Study the drawing (mm; zero at the part's minimum x, y, z) and answer. Round coordinates to 2 decimals unless told otherwise and drop trailing zeros. Order: outer loops, then holes, each group sorted by start corner. A loop starts at its lowest first (then second) coordinate and runs counter-clockwise, first axis right, second up. Notation, with made-up numbers: (-38.5, -1) -> (-12.5, -1) arc R32 ccw to (-12.5, 36) -> close; hole circle Ø8 at (19.25, 7). An arc over 180 degrees is marked (long way). Use one line per item in the form item = value.
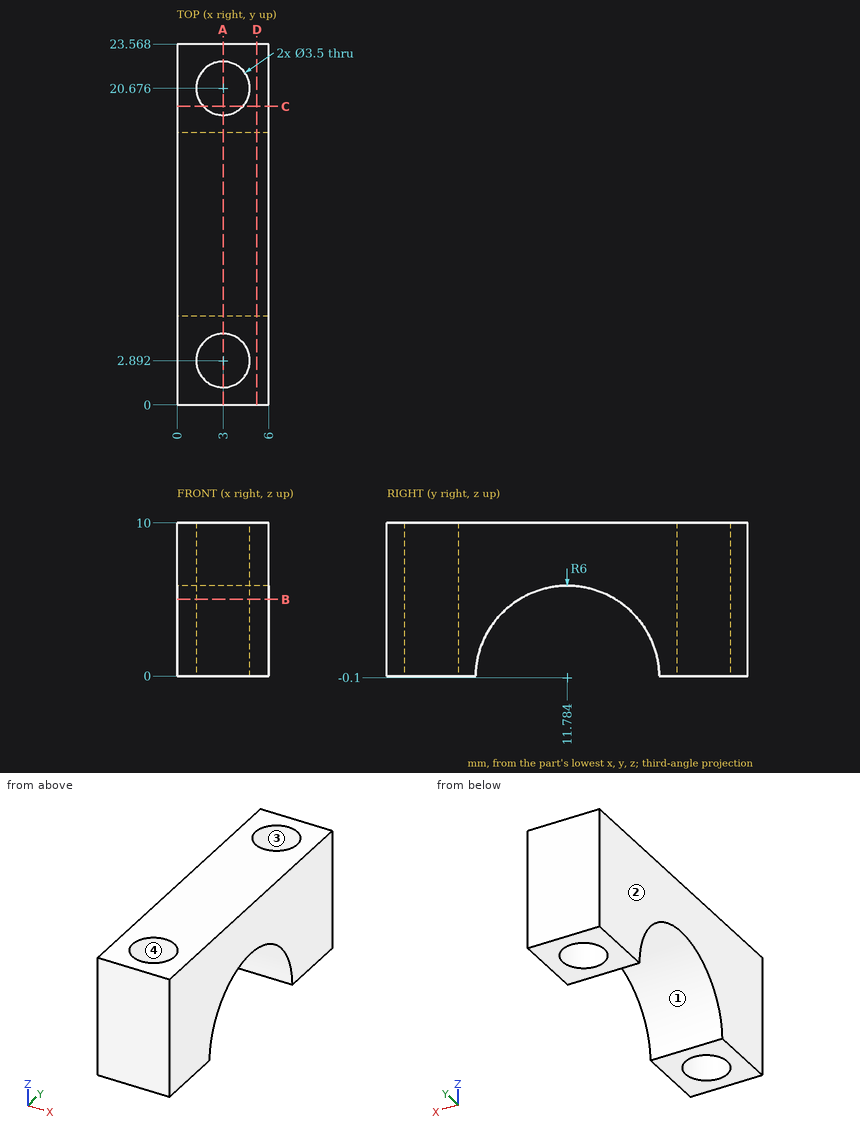
Item 1: The part is cut by section C-C, the plane y = 19.5. Give the vertices of the cut face in (x, z).
Findings:
outline = (0, 0) -> (1.7, 0) -> (1.7, 10) -> (0, 10) -> close; (4.3, 0) -> (6, 0) -> (6, 10) -> (4.3, 10) -> close
Item 2: Consider line 1 along Y through (x, z) = (2.95, 6.75) (1 decimal); line 2 along Y through (x, z) = (3, 2.5) (1 decimal); line 3 along Y through (x, z) = (3, 3.75) (1 decimal). Determine where each line is inside the solid, lowest interval first.
Findings:
line_1 = 0 to 1.1, 4.6 to 18.9, 22.4 to 23.6
line_2 = 0 to 1.1, 4.6 to 6.4, 17.2 to 18.9, 22.4 to 23.6
line_3 = 0 to 1.1, 4.6 to 7.2, 16.4 to 18.9, 22.4 to 23.6
Item 3: A flat-ended cylindrical pin translates along its axis: P1, Ø3, axis at x = 3, y = 20.68, coming from the +Z side. Find the tip coordinate at first contact, or state that the pin passes through.
Findings:
P1 = through
Item 4: The part is cut by section B-B, the plane z = 5. Give the number of separate pieces and of enclosed holes in the cut face.
Findings:
separate_pieces = 2
enclosed_holes = 2
Item 5: The part is cut by section A-A, the plane x = 3. Give the vertices of the cut face in (y, z) (1 decimal), and give its area (3 significant figures).
Findings:
outline = (0, 0) -> (1.1, 0) -> (1.1, 10) -> (0, 10) -> close; (4.6, 0) -> (5.8, 0) arc R6 cw to (17.8, 0) -> (18.9, 0) -> (18.9, 10) -> (4.6, 10) -> close; (22.4, 0) -> (23.6, 0) -> (23.6, 10) -> (22.4, 10) -> close
area = 110 mm^2
Item 6: Determine the mould class of the marked faces 1, 2, 3 and 4 for opening direction X: released by +X, released by -X, zero draft, split by the parting line, or undercut.
Findings:
face_1 = zero draft
face_2 = released by -X
face_3 = undercut
face_4 = undercut
Item 7: The part is cut by section D-D, the plane x = 5.2. Give the vertices of the cut face in (y, z) (1 decimal).
Findings:
outline = (0, 0) -> (5.8, 0) arc R6 cw to (17.8, 0) -> (23.6, 0) -> (23.6, 10) -> (0, 10) -> close
